Build history of the part. All positions in model axes, mm. A direction names the side the tool comes from. Round coordinates to 2 decimals unless told otherwise and drop trailing zeros. Loops run counter-clockwise (first coordinate to the right, second up) from the corner with the lowest first, then second, coordinate; pieces in that order, holes last. Notation, with made-up numbers: (83, 82.25) -> (141, 82.25) arc R24 ccw to (141, 92.25) -> close; hole circle Ø11 at (36, 71.5). An arc over 180 degrees is marked (long way). Put each result on its own line as item: value. Start each with the question number.
```python
from build123d import *

# Parameters (mm, degrees)
SKETCH1_W           = 11.605976064
SKETCH1_H           = 10
SKETCH1_R           = 3
BOSS_EXTRUDE1_DEPTH = 25
SKETCH2_W           = 11.605976064
SKETCH2_H           = 10
BOSS_EXTRUDE2_DEPTH = 2
FILLET1_R           = 5
CUT_EXTRUDE1_DEPTH  = 1.9


with BuildPart() as part:
    # Sketch1 → Boss-Extrude1 (new body)
    with BuildSketch(Plane.XY):
        Rectangle(SKETCH1_W, SKETCH1_H)
        Circle(SKETCH1_R, mode=Mode.SUBTRACT)
    extrude(amount=BOSS_EXTRUDE1_DEPTH)

    # Sketch2 → Boss-Extrude2 (add)
    with BuildSketch(Plane(origin=(0, 0, 0), x_dir=(-1, 0, 0), z_dir=(0, 0, -1))):
        Rectangle(SKETCH2_W, SKETCH2_H)
    extrude(amount=BOSS_EXTRUDE2_DEPTH)

    # Fillet1
    fillet1_edges = [part.edges().sort_by_distance(p)[0] for p in [
        (5.802988032, 0, -2),
        (-5.802988032, 0, -2),
    ]]
    fillet(fillet1_edges, radius=FILLET1_R)

    # Sketch3 → Cut-Extrude1 (cut)
    with BuildSketch(Plane(origin=(0, 5, 0), x_dir=(1, 0, 0), z_dir=(0, 1, 0))):
        with BuildLine():
            Line((3.629140862, -2.424827665), (1.665427656, -20.71398307))
            ThreePointArc((1.665427656, -20.71398307), (0, -22.210165502), (-1.665427656, -20.71398307))
            Line((-1.665427656, -20.71398307), (-3.629140862, -2.424827665))
            ThreePointArc((-3.629140862, -2.424827665), (0, 1.614834498), (3.629140862, -2.424827665))
        make_face()
    extrude(amount=-CUT_EXTRUDE1_DEPTH, mode=Mode.SUBTRACT)


solid = part.part
```
Item 1: Cut at C-C on y = 0. Write the cut outline in (x, z), then the cut area to 3 significant figures.
Item 2: Drop flat-ended pins along their axis: pin 1 (1.8 mm diameter, centred on x = 1, y = -0.5, fed in from +Z); pin 2 (2 mm diameter, centred on x = 1, z = 7.5, fed in from +Y). Give the stop position or say it passes through.
Item 3: 3-axis set-ups, long thin cutter, end or side, ignore diameter. For faces 1 (the face through (0, -5, 12)), 2 (the face through (-3, 0, 12)), 3 (the face through (0.03, 4.06, 22.21)): which of +Z, -Z, +X, -X, +Y, -Y reach the whole face in a straight line?
Item 4: Cut at A-A on x = 0. Write the cut outline in (y, z).
Item 5: Cut at B-B on z = 8.5. Write the cut outline in (x, y).
Item 6: Wall check: line 1 (X direction, y = -2.5, z = 5); line 2 (Z direction, x = 0.5, y = -1.25); line 3 (X direction, y = -1.25, z = 11.75). Give the ranges that are in metal, low to high. Write a range as from..to.
Item 7: Cut at D-D on z = 18. Write the cut outline in (x, y), then the cut area to 3 significant figures.
Item 8: Pull direction Z, two halves, no side cores. Call faces 4 (the face through (3, 5, 15)), 5 (the face through (-0.086, 4.063, -1.614)), 6 (the face through (4.377, 0.07, -0.496)): +Z half, -Z half, draft (parallel to the pull), parting line (faces both ways), or undercut.
Ans:
1. outline: (-5.8, 3) arc R5 ccw to (-0.8, -2) -> (0.8, -2) arc R5 ccw to (5.8, 3) -> (5.8, 25) -> (3, 25) -> (3, 0) -> (-3, 0) -> (-3, 25) -> (-5.8, 25) -> close
1. area: 153 mm2
2. pin 1: stops at z = 0
2. pin 2: stops at y = 3.1
3. face 1: +Z, -Z, +X, -X, -Y
3. face 2: +Z
3. face 3: +Y
4. outline: (-5, -2) -> (5, -2) -> (5, -1.61) -> (3.1, -1.61) -> (3.1, 22.21) -> (5, 22.21) -> (5, 25) -> (3, 25) -> (3, 0) -> (-3, 0) -> (-3, 25) -> (-5, 25) -> close
5. outline: (-5.8, -5) -> (5.8, -5) -> (5.8, 5) -> (2.98, 5) -> (2.98, 3.1) -> (-2.98, 3.1) -> (-2.98, 5) -> (-5.8, 5) -> close; hole circle Ø6 at (0, 0)
6. line 1: x = -5.8..-1.66, 1.66..5.8
6. line 2: z = -2..0
6. line 3: x = -5.8..-2.73, 2.73..5.8
7. outline: (-5.8, -5) -> (5.8, -5) -> (5.8, 5) -> (1.96, 5) -> (1.96, 3.1) -> (-1.96, 3.1) -> (-1.96, 5) -> (-5.8, 5) -> close; hole circle Ø6 at (0, 0)
7. area: 80.3 mm2
8. face 4: draft
8. face 5: undercut
8. face 6: -Z half
